```python
from build123d import *


# Read off the part's stored shape, not the designer's step: Thicken1
with BuildPart() as part:
    # Thicken1 outline → Thicken1 (revolve)
    with BuildSketch(Plane.XY):
        Polygon((43.000126639, 96.3), (31.5, 0), (33.485889655, -0.237154543), (44.986016294, 96.062845457), align=None)
    revolve(axis=Axis((0, 0, 0), (0, 1, 0)))


solid = part.part
```
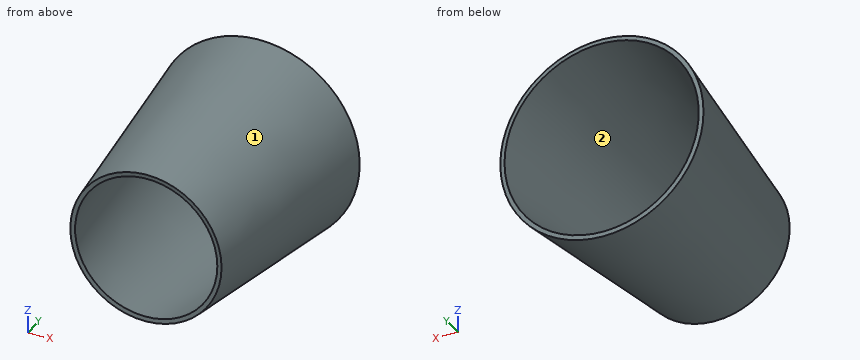
The listing builds one solid part. Answer for the finished solid, in the listing's coordinates (mm). Face numbers are marked on the shaded views. Round coordinates to 2 decimals unless told otherwise and drop trailing zeros. Order: outer loops, then holes, each group sorted by start corner. A loop starts at its lowest first (then second) coordinate and runs counter-clockwise, first axis right, second up. Notation, with made-up numbers: (-3.75, 31.5) -> (24.25, 31.5) arc R19 cw to (24.25, 57.5) -> close; hole circle Ø5 at (72, 11). An arc over 180 degrees is marked (long way). Answer as CSV lines item,"result".
Q1. A cutting plane is placed at B-B on y = 90. Determine the outline of the cut face in (x, z), plus the area to 3 significant figures.
Computed values:
outline,"circle Ø88.52 at (0, 0); hole circle Ø84.5 at (0, 0)"
area,"547 mm^2"
Q2. For a pull along X with two mould halves and no side action, classify the marked faces 1 and 2 as +X half, -X half, draft (parallel to the pull), parting line (faces both ways), or undercut.
Computed values:
face 1,"parting line"
face 2,"undercut"
Q3. Consider line 1 (Z direction, x = 10.5, y = 12); line 2 (Z direction, x = -3, y = 11.5); line 3 (X direction, y = 78.5, z = -31). Determine where each line is inside the solid, lowest interval first. Write a range as from..to.
Computed values:
line 1,"z = -33.33..-31.21, 31.21..33.33"
line 2,"z = -34.76..-32.74, 32.74..34.76"
line 3,"x = -29.64..-26.64, 26.64..29.64"
Q4. A cutting plane is placed at A-A on x = 0. Determine the outline of the cut face in (y, z).
Computed values:
outline,"(-0.24, -33.49) -> (96.06, -44.99) -> (96.3, -43) -> (0, -31.5) -> close; (-0.24, 33.49) -> (0, 31.5) -> (96.3, 43) -> (96.06, 44.99) -> close"
Q5. Given pin 1 (4 mm diameter, centred on x = 26.5, y = 40.5, fed in from -Z); pin 2 (10 mm diameter, centred on y = 58, z = -26.5, fed in from -X); pin 3 (3 mm diameter, centred on x = 8, y = 48.5, fed in from -Z); pin 4 (3 mm diameter, centred on x = 10, z = -26.5, fed in from -Y), each flat-ended and moving along its own axis, determine where each tip first touches the part or whether it passes through.
Computed values:
pin 1,"stops at z = -29.53"
pin 2,"stops at x = -34.33"
pin 3,"stops at z = -38.82"
pin 4,"passes through"
Q6. A cutting plane is placed at C-C on y = 47. Determine the outline of the cut face in (x, z), plus the area to 3 significant figures.
Computed values:
outline,"circle Ø78.25 at (0, 0); hole circle Ø74.23 at (0, 0)"
area,"482 mm^2"
